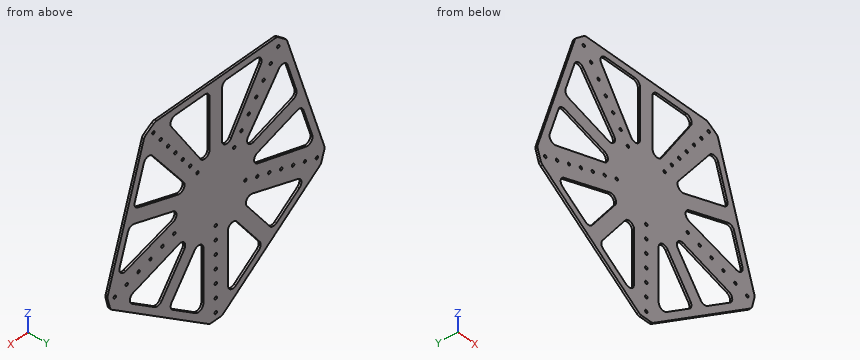
from build123d import *

# Parameters (mm, degrees)
BOSS_EXTRUDE1_DEPTH = 3.81
SKETCH1_R           = 2.54
CUT_EXTRUDE2_DEPTH  = 3.81
CUT_EXTRUDE4_DEPTH  = 25.4
FILLET1_R           = 10
CUT_EXTRUDE5_DEPTH  = 25.4
FILLET2_R           = 10
FILLET3_R           = 10


with BuildPart() as part:
    # Sketch2 → Boss-Extrude1 (new body)
    with BuildSketch(Plane(origin=(0, 0, 0), x_dir=(1, 0, 0), z_dir=(0, 1, 0))):
        Polygon((-214.113347974, 82.923214231), (-222.375187677, 58.900508182), (-144.642224503, -177.47641221), (-125.09137467, -193.780037034), (124.093192846, -192.406157618), (145.640406327, -178.850291626), (221.336035454, 58.562867157), (215.102095915, 83.244477912), (12.7, 229.477457482), (-12.7, 229.477457482), align=None)
    extrude(amount=BOSS_EXTRUDE1_DEPTH)

    # Sketch1 → Cut-Extrude2 (cut)
    with BuildSketch(Plane(origin=(0, 0, 0), x_dir=(1, 0, 0), z_dir=(0, 1, 0))):
        with Locations((108.960749485, 35.403493624)):
            Circle(SKETCH1_R)
        with Locations((84.688009575, 27.516802346)):
            Circle(SKETCH1_R)
        with Locations((82.342824886, -113.335175454)):
            Circle(SKETCH1_R)
        with Locations((97.344203151, -133.98280128)):
            Circle(SKETCH1_R)
        with Locations((127.346959681, -175.278052932)):
            Circle(SKETCH1_R)
        with Locations((-206.051709128, 66.950258738)):
            Circle(SKETCH1_R)
        with Locations((-181.778969217, 59.06356746)):
            Circle(SKETCH1_R)
        with Locations((-157.506229307, 51.176876181)):
            Circle(SKETCH1_R)
        with Locations((-133.233489396, 43.290184903)):
            Circle(SKETCH1_R)
        with Locations((-108.960749485, 35.403493624)):
            Circle(SKETCH1_R)
        with Locations((-84.688009575, 27.516802346)):
            Circle(SKETCH1_R)
        with Locations((-60.415269664, 19.630111067)):
            Circle(SKETCH1_R)
        with Locations((0, 216.655588388)):
            Circle(SKETCH1_R)
        with Locations((0, 191.133719293)):
            Circle(SKETCH1_R)
        with Locations((0, 165.611850198)):
            Circle(SKETCH1_R)
        with Locations((0, 140.089981103)):
            Circle(SKETCH1_R)
        with Locations((0, 114.568112009)):
            Circle(SKETCH1_R)
        with Locations((0, 89.046242914)):
            Circle(SKETCH1_R)
        with Locations((0, 63.524373819)):
            Circle(SKETCH1_R)
        with Locations((206.051709128, 66.950258738)):
            Circle(SKETCH1_R)
        with Locations((181.778969217, 59.06356746)):
            Circle(SKETCH1_R)
        with Locations((157.506229307, 51.176876181)):
            Circle(SKETCH1_R)
        with Locations((133.233489396, 43.290184903)):
            Circle(SKETCH1_R)
        with Locations((37.338690092, -51.392297977)):
            Circle(SKETCH1_R)
        with Locations((52.340068357, -72.039923802)):
            Circle(SKETCH1_R)
        with Locations((67.341446622, -92.687549628)):
            Circle(SKETCH1_R)
        with Locations((112.345581416, -154.630427106)):
            Circle(SKETCH1_R)
        with Locations((-127.346959681, -175.278052932)):
            Circle(SKETCH1_R)
        with Locations((-112.345581416, -154.630427106)):
            Circle(SKETCH1_R)
        with Locations((-97.344203151, -133.98280128)):
            Circle(SKETCH1_R)
        with Locations((-82.342824886, -113.335175454)):
            Circle(SKETCH1_R)
        with Locations((-67.341446622, -92.687549628)):
            Circle(SKETCH1_R)
        with Locations((-52.340068357, -72.039923802)):
            Circle(SKETCH1_R)
        with Locations((-37.338690092, -51.392297977)):
            Circle(SKETCH1_R)
    extrude(amount=CUT_EXTRUDE2_DEPTH, mode=Mode.SUBTRACT)

    # Sketch4 → Cut-Extrude4 (cut)
    with BuildSketch(Plane(origin=(0, 3.81, 0), x_dir=(1, 0, 0), z_dir=(0, 1, 0))):
        Polygon((-45.070854373, 42.218517188), (-116.134569677, 138.509259641), (-186.385554028, 87.392588613), align=None)
    extrude(amount=-CUT_EXTRUDE4_DEPTH, mode=Mode.SUBTRACT)

    # Fillet1
    fillet1_edges = [part.edges().sort_by_distance(p)[0] for p in [
        (-45.070854373, 1.905, -42.218517188),
        (-186.385554028, 1.905, -87.392588613),
        (-116.134569677, 1.905, -138.509259641),
    ]]
    fillet(fillet1_edges, radius=FILLET1_R)

    # Sketch4<3> → Cut-Extrude5 (cut)
    with BuildSketch(Plane(origin=(0, 3.81, 0), x_dir=(1, 0, 0), z_dir=(0, 1, 0))):
        Polygon((-45.070854373, 42.218517188), (-116.134569677, 138.509259641), (-186.385554028, 87.392588613), align=None)
        Polygon((-25.263196152, 204.629928972), (-95.595688183, 153.453950571), (-24.449522239, 57.051488188), align=None)
        Polygon((96.100640401, 153.553690969), (25.4, 204.634018259), (25.4, 57.052227702), align=None)
        Polygon((46.069621628, 42.286739176), (116.689753838, 138.678314353), (187.309886047, 87.656153224), align=None)
        Polygon((-54.313264472, -4.068117885), (-202.740299234, 39.846930078), (-175.394631138, -43.308073239), align=None)
        Polygon((-46.329229165, -27.545327403), (-167.47690719, -67.384952942), (-140.115544314, -150.587682263), align=None)
        Polygon((-12.7, -43.090401677), (-101.684923108, -180.937649266), (-12.7, -180.397220358), align=None)
        Polygon((12.7, -43.122873263), (12.7, -180.257313283), (100.864034479, -179.820968664), align=None)
        Polygon((46.904199543, -26.956649015), (140.994368681, -151.614087132), (168.389811964, -65.690516628), align=None)
        Polygon((56.068689502, -3.218822472), (201.972389344, 39.638494676), (176.105537606, -41.490773287), align=None)
    extrude(amount=-CUT_EXTRUDE5_DEPTH, mode=Mode.SUBTRACT)

    # Fillet2
    fillet2_edges = [part.edges().sort_by_distance(p)[0] for p in [
        (-45.070854373, 1.905, -42.218517188),
        (-186.385554028, 1.905, -87.392588613),
        (-116.134569677, 1.905, -138.509259641),
        (-25.263196152, 1.905, -204.629928972),
        (-24.449522239, 1.905, -57.051488188),
        (-95.595688183, 1.905, -153.453950571),
        (187.309886047, 1.905, -87.656153224),
        (46.069621628, 1.905, -42.286739176),
        (116.689753838, 1.905, -138.678314353),
        (96.100640401, 1.905, -153.553690969),
        (25.4, 1.905, -57.052227702),
        (25.4, 1.905, -204.634018259),
        (-12.7, 1.905, 43.090401677),
        (-12.7, 1.905, 180.397220358),
        (-101.684923108, 1.905, 180.937649266),
        (12.7, 1.905, 43.122873263),
        (100.864034479, 1.905, 179.820968664),
        (12.7, 1.905, 180.257313283),
        (176.105537606, 1.905, 41.490773287),
        (56.068689502, 1.905, 3.218822472),
        (201.972389344, 1.905, -39.638494676),
        (46.904199543, 1.905, 26.956649015),
        (168.389811964, 1.905, 65.690516628),
        (140.994368681, 1.905, 151.614087132),
        (-46.329229165, 1.905, 27.545327403),
        (-140.115544314, 1.905, 150.587682263),
        (-167.47690719, 1.905, 67.384952942),
        (-54.313264472, 1.905, 4.068117885),
        (-175.394631138, 1.905, 43.308073239),
        (-202.740299234, 1.905, -39.846930078),
    ]]
    fillet(fillet2_edges, radius=FILLET2_R)

    # Fillet3
    fillet3_edges = [part.edges().sort_by_distance(p)[0] for p in [
        (-214.113347974, 1.905, -82.923214231),
        (-222.375187677, 1.905, -58.900508182),
        (-144.642224503, 1.905, 177.47641221),
        (-125.09137467, 1.905, 193.780037034),
        (124.093192846, 1.905, 192.406157618),
        (145.640406327, 1.905, 178.850291626),
        (221.336035454, 1.905, -58.562867157),
        (215.102095915, 1.905, -83.244477912),
        (12.7, 1.905, -229.477457482),
        (-12.7, 1.905, -229.477457482),
    ]]
    fillet(fillet3_edges, radius=FILLET3_R)


solid = part.part
Input: part model. Units: mm. Frame: model coordinates. Give positions to 0.01 mm unless a question says otherwise; leave off trailing zeros. Use one line per item in the form item = value. Start each with the question number.
1) Pin query (flat end, axial travel): pin 1 (3 mm diameter, centred on x = 82.34, z = 113.34, fed in from -Y); pin 2 (1 mm diameter, centred on y = 1, z = -57, fed in from -X); pin 3 (1.5 mm diameter, centred on y = 2, z = 36, fed in from -X); pin 4 (1.5 mm diameter, centred on y = 1.5, z = -156, fed in from -X). Return the tip coordinate at first contact, or that it passes through.
2) Section query A-A on y = 2.5. Count the separate pieces of the cut face and the enclosed holes in it, then the cut area to 3 significant figures.
3) Ray query, probe 1 along X at (y, z) = (2.4, 156.5); probe 2 along X at (y, z) = (0.75, 75); probe 3 along Z at (x, y) = (105.5, 0.4). Return the intervals inside material, ascending. Write a range as from..to.
Outcome:
q1.pin_1 = through
q1.pin_2 = -221.74
q1.pin_3 = -191.41
q1.pin_4 = -114.71
q2.separate_pieces = 1
q2.enclosed_holes = 44
q2.area = 81,900 mm^2
q3.probe_1 = -151.54..-114.06, -110.63..-85.91, -12.7..12.7, 85.82..110.63, 114.06..152.77
q3.probe_2 = -178.34..-164.78, -82.5..-33.3, -12.91..12.92, 33.26..83.17, 165.42..178.75
q3.probe_3 = -162.43..-123.41, -61.38..-11.3, 18.98..45.64, 104.59..192.51
